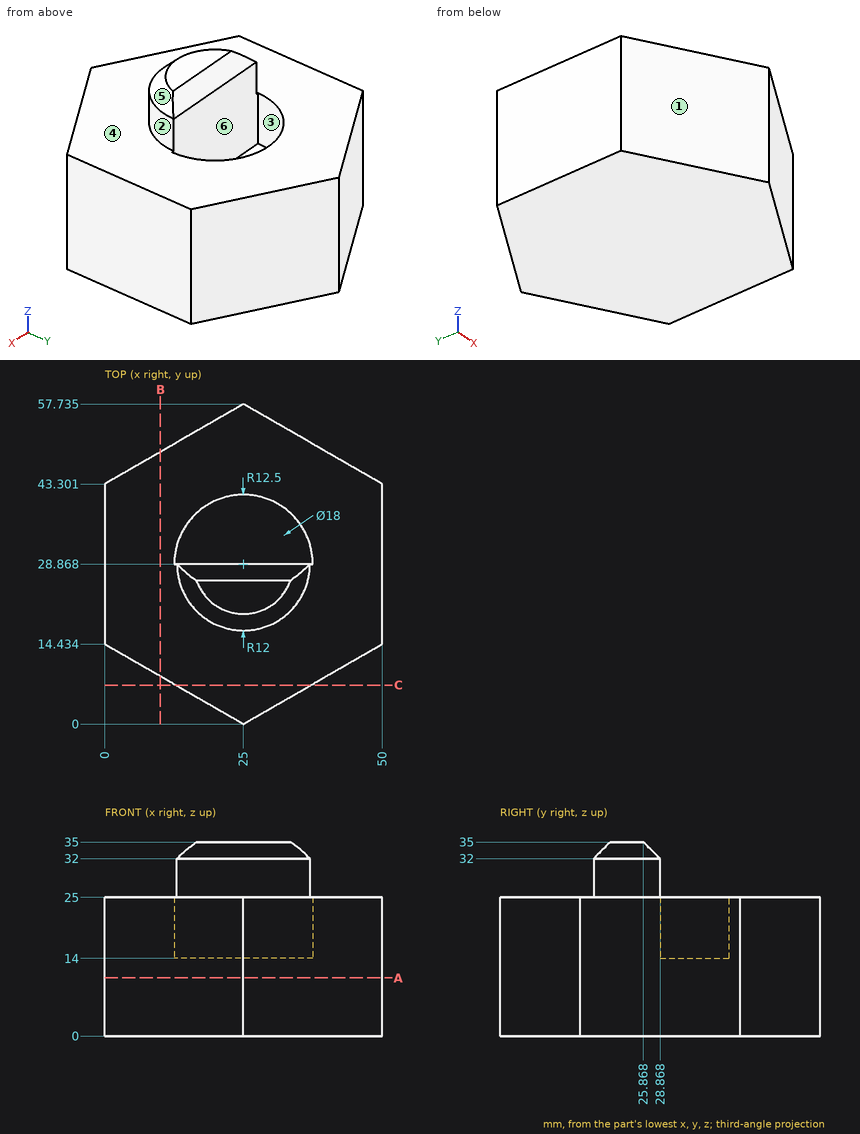
Here's the drawing with two shaded views (mm, measured from the low corner). I have some questions. A direction names the side the tool comes from. Give positions to 0.01 mm unless a question says otherwise; leave off trailing zeros. Order: outer loops, then holes, each group sorted by start corner. A loop starts at its lowest first (then second) coordinate and runs counter-clockwise, first axis right, second up. Notation, with made-up numbers: M 24,4 L 61,4 A17 ccw 61,22 Z; hole C -17,-16.5 d4. An arc over 180 degrees is marked long. One line per question, with ' | ' between items.
Item 1: We'd pull the mould along X, two halves only. Please class the marked faces 4, 5 and 6: released by +X, released by -X, zero draft, split by the parting line, or undercut.
Answer block:
face 4: zero draft | face 5: split by the parting line | face 6: undercut
Item 2: I'm going to push flat-ended pins straight in: pin 1 Ø1.5 at (x, z) = (44.5, 17.5) entering from +Y; pin 2 Ø15 at (x, y) = (21, 15.5) entering from +Z; pin 3 Ø4 at (x, y) = (25, 36.5) entering from +Z; pin 4 Ø12 at (x, y) = (32.5, 13) entering from +Z. Where does each tip first touch, or does it pass through?
Answer block:
pin 1: stops at y = 46.91 | pin 2: stops at z = 35 | pin 3: stops at z = 14 | pin 4: stops at z = 32.45
Item 3: Suppose I cut it at C-C, the plane y = 7. Write out the boundary of the cut face in (x, z) (1 decimal).
Answer block:
outline: M 12.9,0 L 37.1,0 L 37.1,25 L 12.9,25 Z
Item 4: Please list where these lines run through material, in increasing order: L1, parallel to Z at x = 25.5, y = 40; L2, parallel to Z at x = 41, y = 40.5; L3, parallel to Y at x = 22.5, z = 18 (1 decimal).
Answer block:
L1: z = 0 to 14 | L2: z = 0 to 25 | L3: y = 1.4 to 28.9, 41.1 to 56.3
Item 5: Suppose I cut it at A-A, the plane z = 10.5. Write out the boundary of the cut face in (x, y) (1 decimal).
Answer block:
outline: M 0,14.4 L 25,0 L 50,14.4 L 50,43.3 L 25,57.7 L 0,43.3 Z
Item 6: For the marked faces 1, 2 and 3, which set-ups out of +Z, -Z, +X, -X, +Y, -Y let a thin tool reach every point of the face, with its end or its side?
Answer block:
face 1: +Z, -Z, -X, -Y | face 2: +Z, -Y | face 3: +Z
Item 7: Suppose I cut it at B-B, the plane x = 10. Write out the boundary of the cut face in (y, z) (1 decimal).
Answer block:
outline: M 8.7,0 L 49.1,0 L 49.1,25 L 8.7,25 Z
